The drawing under review shows one solid part. Ordinate dimensions are in mm from its lowest x, y, z. Coordinates: 2 decimals unless noted, no trailing zeros. Order: outer loops, then holes, each group sorted by start corner. A loop starts at its lowest first (then second) coordinate and runs counter-clockwise, first axis right, second up. Notation, with made-up numbers: (-0.75, 0.5) -> (37.25, 0.5) arc R21 ccw to (37.25, 25.5) -> close; hole circle Ø11 at (14.25, 69.5). An arc over 180 degrees is marked (long way). Use one line per item in the form item = value.
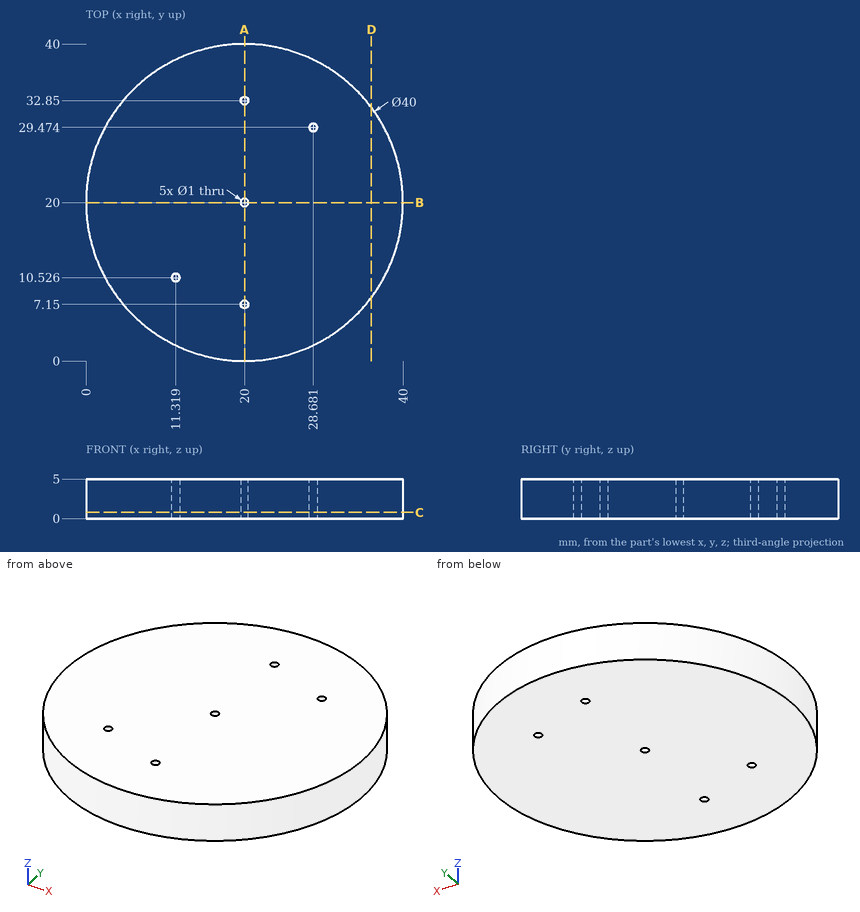
Item 1: We need section C-C (z = 0.8). Write out the cut boundary in (x, y).
Results found:
outline = circle Ø40 at (20, 20); hole circle Ø1 at (11.32, 10.53); hole circle Ø1 at (20, 7.15); hole circle Ø1 at (20, 20); hole circle Ø1 at (20, 32.85); hole circle Ø1 at (28.68, 29.47)
Item 2: Clearance check with flat-ended pins moving along their axes: pin 1 (2 mm diameter, centred on x = 13.5, y = 14, fed in from -Z); pin 2 (1.5 mm diameter, centred on x = 15, z = 4, fed in from -Y); pin 3 (2 mm diameter, centred on y = 6.5, z = 1, fed in from -X); pin 4 (3 mm diameter, centred on x = 24.5, z = 2, fed in from +Y). State where each tip first meets the part, or that it passes through.
Results found:
pin_1 = 0
pin_2 = 0.46
pin_3 = 4.39
pin_4 = 39.77
Item 3: We need section A-A (x = 20). Write out the cut boundary in (y, z).
Results found:
outline = (0, 0) -> (6.65, 0) -> (6.65, 5) -> (0, 5) -> close; (7.65, 0) -> (19.5, 0) -> (19.5, 5) -> (7.65, 5) -> close; (20.5, 0) -> (32.35, 0) -> (32.35, 5) -> (20.5, 5) -> close; (33.35, 0) -> (40, 0) -> (40, 5) -> (33.35, 5) -> close
Item 4: We need section D-D (x = 36). Write out the cut boundary in (y, z), plus the area to 3 significant figures.
Results found:
outline = (8, 0) -> (32, 0) -> (32, 5) -> (8, 5) -> close
area = 120 mm²
Item 5: To check wall thickness, follow L1, parallel to Y at x = 20, z = 1.8; L2, parallel to X at y = 33, z = 3; L3, parallel to Y at x = 21, z = 1.4 (1 decimal). State the ranges of each line that lie inside material, in increasing order. Write a range as from..to.
Results found:
L1 = 0..6.65, 7.65..19.5, 20.5..32.35, 33.35..40
L2 = 4.8..19.52, 20.48..35.2
L3 = 0..40
Item 6: We need section B-B (y = 20). Write out the cut boundary in (x, z).
Results found:
outline = (0, 0) -> (19.5, 0) -> (19.5, 5) -> (0, 5) -> close; (20.5, 0) -> (40, 0) -> (40, 5) -> (20.5, 5) -> close
